```python
from build123d import *

# Parameters (mm, degrees)
BOSS_EXTRUDE1_DEPTH = 30
CUT_EXTRUDE7_DEPTH  = 20
SKETCH5_W           = 17.5
SKETCH5_H           = 10
BOSS_EXTRUDE2_DEPTH = 5
SKETCH6_W           = 40
SKETCH6_H           = 50
BOSS_EXTRUDE3_DEPTH = 30
SKETCH7_W           = 37.5
SKETCH7_H           = 5
CUT_EXTRUDE11_DEPTH = 15
SKETCH8_W           = 37.5
SKETCH8_H           = 5
CUT_EXTRUDE12_DEPTH = 15
CUT_EXTRUDE13_DEPTH = 10
SKETCH10_R          = 15
BOSS_EXTRUDE4_DEPTH = 7.5
SKETCH11_R          = 10
CUT_EXTRUDE14_DEPTH = 7.5
SKETCH12_R          = 5
CUT_EXTRUDE15_DEPTH = 153.5
BOSS_EXTRUDE5_DEPTH = 30
SKETCH14_W          = 17.5
SKETCH14_H          = 10
BOSS_EXTRUDE6_DEPTH = 5
CUT_EXTRUDE16_DEPTH = 20
CUT_EXTRUDE17_DEPTH = 10


with BuildPart() as part:
    # Sketch1 → Boss-Extrude1 (new body)
    with BuildSketch(Plane.XY):
        Polygon((-15, -5), (-7.5, -5), (-7.5, 0), (0, 0), (0, 50), (-7.5, 50), (-7.5, 55), (-15, 55), align=None)
    extrude(amount=BOSS_EXTRUDE1_DEPTH)

    # Sketch3 → Cut-Extrude7 (cut)
    with BuildSketch(Plane(origin=(0, 0, 0), x_dir=(-1, 0, 0), z_dir=(0, 0, -1))):
        with BuildLine():
            Line((15, 35), (15, 15))
            ThreePointArc((15, 15), (5, 25), (15, 35))
        make_face()
    extrude(amount=-CUT_EXTRUDE7_DEPTH, mode=Mode.SUBTRACT)

    # Sketch5 → Boss-Extrude2 (add)
    with BuildSketch(Plane(origin=(0, 50, 0), x_dir=(1, 0, 0), z_dir=(0, 1, 0))):
        with Locations((1.25, -5)):
            Rectangle(SKETCH5_W, SKETCH5_H)
    extrude(amount=BOSS_EXTRUDE2_DEPTH)

    # Sketch6 → Boss-Extrude3 (add)
    with BuildSketch(Plane(origin=(0, 0, 0), x_dir=(-1, 0, 0), z_dir=(0, 0, -1))):
        with Locations((-20, 25)):
            Rectangle(SKETCH6_W, SKETCH6_H)
    extrude(amount=-BOSS_EXTRUDE3_DEPTH)

    # Sketch7 → Cut-Extrude11 (cut)
    with BuildSketch(Plane.XY.offset(30)):
        with Locations((21.25, 47.5)):
            Rectangle(SKETCH7_W, SKETCH7_H)
    extrude(amount=-CUT_EXTRUDE11_DEPTH, mode=Mode.SUBTRACT)

    # Sketch8 → Cut-Extrude12 (cut)
    with BuildSketch(Plane.XY.offset(30)):
        with Locations((21.25, 2.5)):
            Rectangle(SKETCH8_W, SKETCH8_H)
    extrude(amount=-CUT_EXTRUDE12_DEPTH, mode=Mode.SUBTRACT)

    # Sketch9 → Cut-Extrude13 (cut)
    with BuildSketch(Plane.XY.offset(30)):
        with BuildLine():
            Line((-15, 10), (-15, 40))
            ThreePointArc((-15, 40), (0, 25), (-15, 10))
        make_face()
    extrude(amount=-CUT_EXTRUDE13_DEPTH, mode=Mode.SUBTRACT)

    # Sketch10 → Boss-Extrude4 (add)
    with BuildSketch(Plane.XY.offset(30)):
        with Locations((20, 25)):
            Circle(SKETCH10_R)
    extrude(amount=BOSS_EXTRUDE4_DEPTH)

    # Sketch11 → Cut-Extrude14 (cut)
    with BuildSketch(Plane.XY.offset(37.5)):
        with Locations((20, 25)):
            Circle(SKETCH11_R)
    extrude(amount=-CUT_EXTRUDE14_DEPTH, mode=Mode.SUBTRACT)

    # Sketch12 → Cut-Extrude15 (cut)
    with BuildSketch(Plane.XY.offset(30)):
        with Locations((20, 25)):
            Circle(SKETCH12_R)
    extrude(amount=-CUT_EXTRUDE15_DEPTH, mode=Mode.SUBTRACT)

    # Sketch13 → Boss-Extrude5 (add)
    with BuildSketch(Plane.XY.offset(30)):
        Polygon((55, -5), (47.5, -5), (47.5, 0), (40, 0), (40, 50), (47.5, 50), (47.5, 55), (55, 55), align=None)
    extrude(amount=-BOSS_EXTRUDE5_DEPTH)

    # Sketch14 → Boss-Extrude6 (add)
    with BuildSketch(Plane(origin=(0, 50, 0), x_dir=(1, 0, 0), z_dir=(0, 1, 0))):
        with Locations((38.75, -5)):
            Rectangle(SKETCH14_W, SKETCH14_H)
    extrude(amount=BOSS_EXTRUDE6_DEPTH)

    # Sketch15 → Cut-Extrude16 (cut)
    with BuildSketch(Plane(origin=(0, 0, 0), x_dir=(-1, 0, 0), z_dir=(0, 0, -1))):
        with BuildLine():
            Line((-55, 35), (-55, 15))
            ThreePointArc((-55, 15), (-45, 25), (-55, 35))
        make_face()
    extrude(amount=-CUT_EXTRUDE16_DEPTH, mode=Mode.SUBTRACT)

    # Sketch16 → Cut-Extrude17 (cut)
    with BuildSketch(Plane.XY.offset(30)):
        with BuildLine():
            Line((55, 10), (55, 40))
            ThreePointArc((55, 40), (40, 25), (55, 10))
        make_face()
    extrude(amount=-CUT_EXTRUDE17_DEPTH, mode=Mode.SUBTRACT)


solid = part.part
```
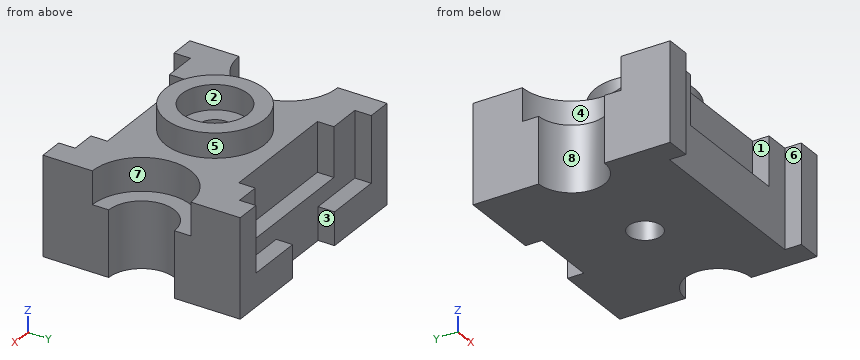
Geometry: final body of the model. Coordinates: model frame, mm. Face numbers are marked on the shaded views. A direction names the side the tool comes from. Coordinates: 2 decimals unless noted, no trailing zeros. Write each loop counter-clockwise with the first axis right and the second up, starting at its lowest first coordinate (ties: lowest second). Pieces come first, ordered by that corner, then holes. Notation, with made-up numbers: M -3.5,-24 L 39.5,-24 A36 cw 39.5,10 Z; hole C 14.25,89 d3. An arc over 180 degrees is marked long. Answer as CSV lines item,"result". Start each with the question number.
Q1. Mould query, pull axis X, two halves, no side actions, for the marked faces 5, 6, 7 and 8. Classes: released by +X, released by -X, zero draft, split by the parting line, or undercut.
Q2. Cut plane C-C on x = 20. Return the cut outline in (y, z), then the cut area to 4 significant figures.
Q3. Pin query (flat end, axial travel): P1, Ø5, axis at y = 33, z = 32, coming from the +X side; P2, Ø4.5, axis at x = 13.5, z = 26, coming from the -Y side; P3, Ø12, axis at y = 32, z = 13, coming from the -X side; P4, Ø10, axis at x = 4.5, z = 9.5, coming from the -Y side. Return the tip coordinate at first contact, or that it passes through.
Q4. Cut plane D-D on y = 2. Return the cut outline in (x, z), then the cut area to 3 significant figures.
Q5. Cut plane B-B on z = 13.5. Return the cut outline in (x, y), then the cut area to 3 significant figures.
Q6. Reachability of the marked faces 1, 2, 3 and 4 from +Z, -Z, +X, -X, +Y, -Y: full face, straight path, thin tool, end or side. Return the list, or none.
Q7. Cut plane A-A on y = 25. Return the cut outline in (x, z), then the cut area to 4 significant figures.
Q8. Line query: line 1 (Y direction, x = 20, z = 32.75); line 2 (X direction, y = -2, z = 3); line 3 (Y direction, x = 20, z = 11.5). Output: solid intervals per line, ascending. Write a range as from..to.
Findings below:
1,face 5,"split by the parting line"
1,face 6,"undercut"
1,face 7,"released by +X"
1,face 8,"released by -X"
2,outline,"M 0,0 L 20,0 L 20,30 L 15,30 L 15,37.5 L 10,37.5 L 10,30 L 5,30 L 5,15 L 0,15 Z; M 30,0 L 50,0 L 50,15 L 45,15 L 45,30 L 40,30 L 40,37.5 L 35,37.5 L 35,30 L 30,30 Z"
2,area,"1,125 mm2"
3,P1,"stops at x = 43.39"
3,P2,"stops at y = 5"
3,P3,"stops at x = -15"
3,P4,"stops at y = 0"
4,outline,"M -15,0 L 55,0 L 55,30 L 40,30 L 40,15 L 2.5,15 L 2.5,30 L -15,30 Z"
4,area,"1,540 mm2"
5,outline,"M -15,-5 L -7.5,-5 L -7.5,0 L 47.5,0 L 47.5,-5 L 55,-5 L 55,15 A10 cw 55,35 L 55,55 L 47.5,55 L 47.5,50 L -7.5,50 L -7.5,55 L -15,55 L -15,35 A10 cw -15,15 Z; hole C 20,25 d10"
5,area,"3,260 mm2"
6,face 1,"+Z, -Y"
6,face 2,"+Z"
6,face 3,"+Z, -Z, +Y"
6,face 4,"+Z, -X"
7,outline,"M -5,0 L 15,0 L 15,30 L 10,30 L 10,37.5 L 5,37.5 L 5,30 L 0,30 L 0,20 L -5,20 Z; M 25,0 L 45,0 L 45,20 L 40,20 L 40,30 L 35,30 L 35,37.5 L 30,37.5 L 30,30 L 25,30 Z"
7,area,"1,175 mm2"
8,line 1,"y = 10..15, 35..40"
8,line 2,"x = -15..-7.5, 47.5..55"
8,line 3,"y = 0..20, 30..50"
